Geometry: final body of the model. Coordinates: model frame, mm. A direction names the side the tool comes from. Give positions to 0.01 mm unless a question says otherwise; leave off trailing zeros. Loops run counter-clockwise (first coordinate to the right, second up) from the corner with the lowest first, then second, coordinate; pieces in that order, holes last.
from build123d import *

# Parameters (mm, degrees)
F0_W     = 70
F0_H     = 50
F1_DEPTH = 4


with BuildPart() as f1:
    # F0 (on Front) → F1 (new body)
    with BuildSketch(Plane.XZ):
        with Locations((35, -25)):
            Rectangle(F0_W, F0_H)
        with BuildLine():
            ThreePointArc((10, -11), (10.87868, -8.87868), (13, -8))
            Line((13, -8), (25.253979, -8))
            Line((25.253979, -8), (25.253979, -16))
            ThreePointArc((25.253979, -16), (32.253979, -23), (39.253979, -16))
            Line((39.253979, -16), (39.253979, -8))
            Line((39.253979, -8), (57, -8))
            ThreePointArc((57, -8), (59.12132, -8.87868), (60, -11))
            Line((60, -11), (60, -35))
            Line((60, -35), (53, -42))
            Line((53, -42), (39.253979, -42))
            Line((39.253979, -42), (39.253979, -34))
            ThreePointArc((39.253979, -34), (32.253979, -27), (25.253979, -34))
            Line((25.253979, -34), (25.253979, -42))
            Line((25.253979, -42), (14, -42))
            ThreePointArc((14, -42), (11.171573, -40.828427), (10, -38))
            Line((10, -38), (10, -11))
        make_face(mode=Mode.SUBTRACT)
    extrude(amount=-F1_DEPTH)


solid = f1.part
Item 1: Section query C-C on y = 0.95. Return loops of the section in (x, z), plus the area to 3 significant figures.
Values follow:
outline: (0, -50) - (70, -50) - (70, 0) - (0, 0) - close; hole (10, -38) arc R4 ccw to (14, -42) - (25.25, -42) - (25.25, -34) arc R7 cw to (39.25, -34) - (39.25, -42) - (53, -42) - (60, -35) - (60, -11) arc R3 ccw to (57, -8) - (39.25, -8) - (39.25, -16) arc R7 cw to (25.25, -16) - (25.25, -8) - (13, -8) arc R3 ccw to (10, -11) - close
area: 2,210 mm2
Item 2: Set-up query: faces 4 (the face through (19, 2, -8)), 5 (the face through (35, 0, -19)). Return all of +Z, -Z, +X, -X, +Y, -Y with unobstructed straight access to the full face (end or side cutting, diameter ignored); none if empty.
Values follow:
face 4: +Y, -Y
face 5: +Z, -Z, +X, -X, -Y
Item 3: Draft query along Z for faces 1 (the face through (0, 2, -25)), 2 (the face through (32.1, 2, -23)), 3 (the face through (35, 2, 0)). Return one class per face: +Z half, -Z half, draft (parallel to the pull), parting line (faces both ways), or undercut.
Values follow:
face 1: draft
face 2: undercut
face 3: +Z half
Item 4: Pin query (flat end, axial travel): pin 1 (8 mm diameter, centred on x = 12, z = -16, fed in from +Y). Return the tip coordinate at first contact, or that it passes through.
Values follow:
pin 1: stops at y = 4
Item 5: Ray query, probe 1 along X at (y, z) = (0.4, -15.5); probe 2 along X at (y, z) = (3.55, -38); probe 3 along Z at (x, y) = (24, 1.25). Return the intervals inside material, ascending.
Values follow:
probe 1: x = 0 to 10, 25.25 to 39.25, 60 to 70
probe 2: x = 0 to 10, 25.25 to 39.25, 57 to 70
probe 3: z = -50 to -42, -8 to 0
Item 6: Section query B-B on x = 21. Return loops of the section in (y, z), plus the area to 3 significant figures.
Values follow:
outline: (0, -50) - (4, -50) - (4, -42) - (0, -42) - close; (0, -8) - (4, -8) - (4, 0) - (0, 0) - close
area: 64.0 mm2
Item 7: Section query A-A on z = -36. Return loops of the section in (x, y), plus the area to 3 significant figures.
Values follow:
outline: (0, 0) - (10, 0) - (10, 4) - (0, 4) - close; (25.25, 0) - (39.25, 0) - (39.25, 4) - (25.25, 4) - close; (59, 0) - (70, 0) - (70, 4) - (59, 4) - close
area: 140 mm2
Item 8: Section query D-D on x = 59. Return loops of the section in (y, z), plus the area to 3 significant figures.
Values follow:
outline: (0, -50) - (4, -50) - (4, -36) - (0, -36) - close; (0, -8.76) - (4, -8.76) - (4, 0) - (0, 0) - close
area: 91.1 mm2
